Design review of the part shown in the three views and the two pictorial views. Dimensions are in mm from the part's minimum x, y and z. A direction names the side the tool comes from. Round coordinates to 2 decimals unless told otherwise and drop trailing zeros. Loops run counter-clockwise (first coordinate to the right, second up) from the corner with the lowest first, then second, coordinate; pieces in that order, holes last.
1. Tool access review of the marked faces 1 and 2: name each direction out of +Z, -Z, +X, -X, +Y, -Y from which nothing blocks a thin tool from reaching the whole face with its end or side.
2. Consider section D-D on y = 95.5. State the section outline as (x, z) points.
3. Consider section C-C on z = 21. State the section outline as (x, y) points, then the cut area to 3 significant figures.
4. Consider section A-A on x = 50.8. State the section outline as (y, z) points, then the cut area to 3 significant figures.
5. To check wall thickness, follow line 1 along Y through (x, z) = (50.5, 37); line 2 along Z through (x, y) = (48.5, 6.5); line 3 along Z through (x, y) = (96, 38.5). State the ranges of each line that lie inside material, in increasing order.
6. Clearance check with flat-ended pins moving along their axes: pin 1 Ø1.5 at (y, z) = (52.5, 24) entering from +X; pin 2 Ø1 at (y, z) = (83.5, 9) entering from +X; pin 3 Ø5 at (x, z) = (80, 19.5) entering from +Y. State where each tip first meets the part, or that it passes through.
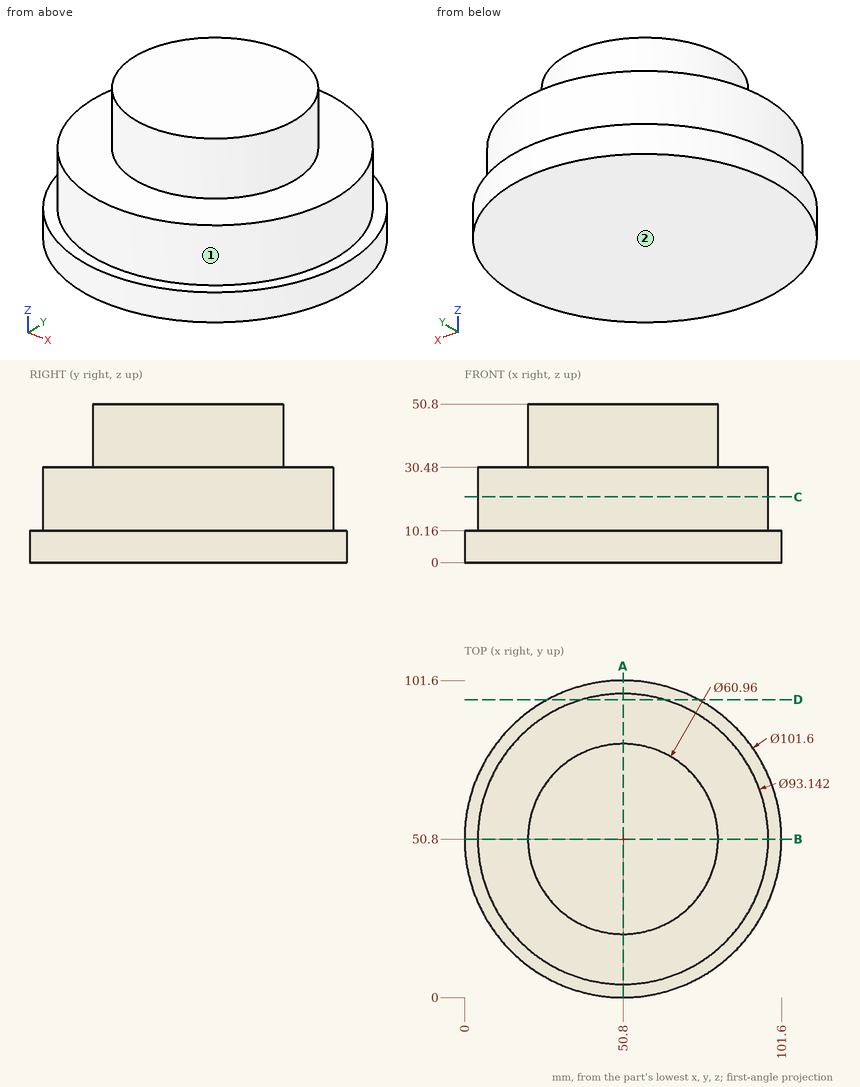
Resolved:
1. face 1: +Z
1. face 2: -Z, +X, -X, +Y, -Y
2. outline: (26.66, 0) - (74.94, 0) - (74.94, 10.16) - (63.87, 10.16) - (63.87, 30.48) - (37.73, 30.48) - (37.73, 10.16) - (26.66, 10.16) - close
3. outline: circle Ø93.14 at (50.8, 50.8)
3. area: 6,810 mm2
4. outline: (0, 0) - (101.6, 0) - (101.6, 10.16) - (97.37, 10.16) - (97.37, 30.48) - (81.28, 30.48) - (81.28, 50.8) - (20.32, 50.8) - (20.32, 30.48) - (4.23, 30.48) - (4.23, 10.16) - (0, 10.16) - close
4. area: 4,160 mm2
5. line 1: y = 20.32 to 81.28
5. line 2: z = 0 to 30.48
5. line 3: z = 0 to 10.16
6. pin 1: stops at x = 97.36
6. pin 2: stops at x = 90.09
6. pin 3: stops at y = 88.96
